from build123d import *

# Parameters (mm, degrees)
SKETCH1_R                                           = 5
SKETCH1_R_2                                         = 4.5
BOSS_EXTRUDE2_DEPTH                                 = 5
CSK_FOR_M3_COUNTERSUNK_FLAT_HEAD_SCREW2_D           = 3.4
CSK_FOR_M3_COUNTERSUNK_FLAT_HEAD_SCREW2_CSINK_D     = 6.3
CSK_FOR_M3_COUNTERSUNK_FLAT_HEAD_SCREW2_CSINK_ANGLE = 90
CIRPATTERN2_COUNT                                   = 4
M2_TAPPED_HOLE1_D                                   = 1.6
M2_TAPPED_HOLE1_DEPTH                               = 5
M2_TAPPED_HOLE1_TIP                                 = 0.480688495
M2_TAPPED_HOLE2_D                                   = 1.6
M2_TAPPED_HOLE2_DEPTH                               = 5
M2_TAPPED_HOLE2_TIP                                 = 0.480688495


with BuildPart() as part:
    # Sketch1 → Boss-Extrude2 (new body)
    with BuildSketch(Plane(origin=(0, 0, 0), x_dir=(1, 0, 0), z_dir=(0, 1, 0))):
        Polygon((-37.002207947, 0), (-37.002207947, 15), (42.997792053, 15), (42.997792053, -15), (-37.002207947, -15), align=None)
        with Locations(Location((-25, 0, 0), (0, 0, 270))):
            Circle(SKETCH1_R, mode=Mode.SUBTRACT)
        with Locations(Location((25, 0, 0), (0, 0, 270))):
            Circle(SKETCH1_R_2, mode=Mode.SUBTRACT)
    extrude(amount=BOSS_EXTRUDE2_DEPTH)

    # CSK for M3 Countersunk Flat Head Screw2 (through all)
    with Locations(Plane(origin=(0, 5, 0), x_dir=(1, 0, 0), z_dir=(0, 1, 0))):
        with Locations((14, 0)):
            csk_for_m3_countersunk_flat_head_screw2 = CounterSinkHole(CSK_FOR_M3_COUNTERSUNK_FLAT_HEAD_SCREW2_D / 2, CSK_FOR_M3_COUNTERSUNK_FLAT_HEAD_SCREW2_CSINK_D / 2, counter_sink_angle=CSK_FOR_M3_COUNTERSUNK_FLAT_HEAD_SCREW2_CSINK_ANGLE)

    # CirPattern2: CSK for M3 Countersunk Flat Head Screw2 ×4 about axis
    cirpattern2_axis = Axis((25, 0, 0), (0, 1, 0))
    for i in range(1, CIRPATTERN2_COUNT):
        add(csk_for_m3_countersunk_flat_head_screw2.rotate(cirpattern2_axis, i * 360 / CIRPATTERN2_COUNT), mode=Mode.SUBTRACT)

    # M2 Tapped Hole1
    with Locations(Plane.XY.offset(15)):
        with Locations((15.997792053, 2.5), (33.997792053, 2.5)):
            Hole(M2_TAPPED_HOLE1_D / 2, depth=M2_TAPPED_HOLE1_DEPTH)
            with Locations((0, 0, -(M2_TAPPED_HOLE1_DEPTH + M2_TAPPED_HOLE1_TIP / 2))):  # 118° drill point
                Cone(0, M2_TAPPED_HOLE1_D / 2, M2_TAPPED_HOLE1_TIP, mode=Mode.SUBTRACT)

    # M2 Tapped Hole2
    with Locations(Plane(origin=(0, 0, -15), x_dir=(-1, 0, 0), z_dir=(0, 0, -1))):
        with Locations((-33.997792053, 2.5), (-15.997792053, 2.5)):
            Hole(M2_TAPPED_HOLE2_D / 2, depth=M2_TAPPED_HOLE2_DEPTH)
            with Locations((0, 0, -(M2_TAPPED_HOLE2_DEPTH + M2_TAPPED_HOLE2_TIP / 2))):  # 118° drill point
                Cone(0, M2_TAPPED_HOLE2_D / 2, M2_TAPPED_HOLE2_TIP, mode=Mode.SUBTRACT)


solid = part.part
Input: part model. Units: mm. Frame: model coordinates. A direction names the side the tool comes from. Give positions to 0.01 mm unless a question says otherwise; leave off trailing zeros. Order: outer loops, then holes, each group sorted by start corner. A loop starts at its lowest first (then second) coordinate and runs counter-clockwise, first axis right, second up. Notation, with made-up numbers: (52.25, -18.5) - (68.25, -18.5) arc R9 cw to (68.25, -3.5) - close; hole circle Ø10 at (31.25, 75.5). An arc over 180 degrees is marked (long way). Write each question's results on one line, items separated by ' | '.
Item 1: Section A-A (x = 25). Return loops of the section in (y, z).
A:
outline: (0, -15) - (5, -15) - (5, -14.15) - (3.55, -12.7) - (0, -12.7) - close; (0, -9.3) - (3.55, -9.3) - (5, -7.85) - (5, -4.5) - (0, -4.5) - close; (0, 4.5) - (5, 4.5) - (5, 7.85) - (3.55, 9.3) - (0, 9.3) - close; (0, 12.7) - (3.55, 12.7) - (5, 14.15) - (5, 15) - (0, 15) - close
Item 2: Material intervals for line 1 along X through (y, z) = (2.5, 12.75); line 2 along X through (y, z) = (0.85, 9.5); line 3 along X through (y, z) = (1.15, 11), sorted ascending.
A:
line 1: x = -37 to 15.2, 16.8 to 33.2, 34.8 to 43 | line 2: x = -37 to 24.2, 25.8 to 43 | line 3: x = -37 to 23.3, 26.7 to 43
Item 3: Contact query for flat-ended pins moving along their axis: pin 1 Ø1.4 at (x, y) = (16, 2.5) entering from -Z; pin 2 Ø2.5 at (x, z) = (36, 0) entering from -Y; pin 3 Ø1.4 at (x, y) = (34, 2.5) entering from +Z; pin 4 Ø4.5 at (x, z) = (25, 11) entering from +Y. Output: stop coordinate, or through.
A:
pin 1: stops at z = -9.94 | pin 2: passes through | pin 3: stops at z = 9.94 | pin 4: stops at y = 4.1
Item 4: Section D-D (x = 36). Return loops of the section in (y, z), and give its area (3 significant figures).
A:
outline: (0, -15) - (5, -15) - (5, -3.15) - (3.55, -1.7) - (0, -1.7) - close; (0, 1.7) - (3.55, 1.7) - (5, 3.15) - (5, 15) - (0, 15) - close | area: 131 mm^2
Item 5: Section C-C (y = 1). Return loops of the section in (x, z).
A:
outline: (-37, -15) - (43, -15) - (43, 15) - (-37, 15) - close; hole circle Ø10 at (-25, 0); hole circle Ø3.4 at (14, 0); hole circle Ø9 at (25, 0); hole circle Ø3.4 at (25, -11); hole circle Ø3.4 at (25, 11); hole circle Ø3.4 at (36, 0)
Item 6: Section B-B (z = 11). Return loops of the section in (x, y).
A:
outline: (-37, 0) - (23.3, 0) - (23.3, 3.55) - (21.85, 5) - (-37, 5) - close; (26.7, 0) - (43, 0) - (43, 5) - (28.15, 5) - (26.7, 3.55) - close; hole circle Ø1.6 at (16, 2.5); hole circle Ø1.6 at (34, 2.5)
Item 7: Draft query along Z for faces 3 (the cylindrical face through (12.43, 1.75, 0.65)), 4 (the conical face through (16.13, 2.54, 9.6)), 5 (the conical face through (15.87, 2.45, -9.6)), 6 (the flat face through (4, 0, 0)). Return one class per face: released by +Z, released by -Z, zero draft, split by the parting line, or undercut.
A:
face 3: undercut | face 4: released by +Z | face 5: released by -Z | face 6: zero draft
Item 8: Access query for faces 1 (the conical face through (33.86, 2.51, 9.6)), 2 (the cylindrical face through (34.76, 2.74, -12.46)). Directions: +Z, -Z, +X, -X, +Y, -Y. A direction counts if a zero-diameter tool reaches every point of the face in a straight line with its end or side. Return the directions, or none.
A:
face 1: +Z | face 2: -Z
